from build123d import *

# Parameters (mm, degrees)
SKETCH1_R               = 15
SKETCH1_R_2             = 3
BOSS_EXTRUDE1_DEPTH     = 10
SKETCH2_W               = 15
SKETCH2_H               = 30
BOSS_EXTRUDE2_DEPTH     = 10
FILLET1_R               = 15
SKETCH5_W               = 10
SKETCH5_H               = 2
BOSS_EXTRUDE3_DEPTH     = 10
BOSS_EXTRUDE4_START     = -3
SKETCH7_R               = 3
BOSS_EXTRUDE4_DEPTH     = 3
CHAMFER1_SIZE           = 0.7
BOSS_EXTRUDE6_DEPTH     = 10
FILLET4_R               = 2
FILLET2_R               = 10
CUT_EXTRUDE1_DEPTH      = 63.556116013
CUT_EXTRUDE1_DEPTH_BACK = 63.556116013
SKETCH10_R              = 1.25
SKETCH11_R              = 9.5
SKETCH11_R_2            = 6
CUT_EXTRUDE2_DEPTH      = 5


with BuildPart() as part:
    # Sketch1 → Boss-Extrude1 (new body)
    with BuildSketch(Plane.XY):
        Circle(SKETCH1_R)
        Circle(SKETCH1_R_2, mode=Mode.SUBTRACT)
    extrude(amount=BOSS_EXTRUDE1_DEPTH)

    # Sketch2 → Boss-Extrude2 (add)
    with BuildSketch(Plane.XY):
        with Locations((0, 27.990381057)):
            Rectangle(SKETCH2_W, SKETCH2_H)
    extrude(amount=BOSS_EXTRUDE2_DEPTH)

    # Fillet1
    fillet1_edges = [part.edges().sort_by_distance(p)[0] for p in [
        (-7.5, 12.990381057, 5),
        (7.5, 12.990381057, 5),
    ]]
    fillet(fillet1_edges, radius=FILLET1_R)

    # Sketch5 → Boss-Extrude3 (add)
    with BuildSketch(Plane(origin=(0, 0, 0), x_dir=(-1, 0, 0), z_dir=(0, 0, -1))):
        with Locations((0, 2.5)):
            Rectangle(SKETCH5_W, SKETCH5_H)
    extrude(amount=-BOSS_EXTRUDE3_DEPTH)

    # Sketch7 → Boss-Extrude4 (add)
    with BuildSketch(Plane.XY.offset(10).offset(BOSS_EXTRUDE4_START)):
        Circle(SKETCH7_R)
    extrude(amount=BOSS_EXTRUDE4_DEPTH)

    # Chamfer1
    chamfer1_edges = [part.edges().sort_by_distance(p)[0] for p in [
        (0, 1.5, 7),
        (0, -3, 7),
    ]]
    chamfer(chamfer1_edges, length=CHAMFER1_SIZE)

    # Sketch9 → Boss-Extrude6 (add)
    with BuildSketch(Plane(origin=(0, 0, 0), x_dir=(-1, 0, 0), z_dir=(0, 0, -1))):
        with BuildLine():
            Line((-15, 53.990381057), (-15, 50.490381057))
            ThreePointArc((-15, 50.490381057), (-12.803300859, 45.187080198), (-7.5, 42.990381057))
            Line((-7.5, 42.990381057), (0, 42.990381057))
            Line((0, 42.990381057), (0, 46.490381057))
            Line((0, 46.490381057), (-7.5, 46.490381057))
            ThreePointArc((-7.5, 46.490381057), (-10.328427125, 47.661953932), (-11.5, 50.490381057))
            Line((-11.5, 50.490381057), (-11.5, 53.990381057))
            Line((-11.5, 53.990381057), (-15, 53.990381057))
        make_face()
        with BuildLine():
            Line((0, 46.490381057), (0, 42.990381057))
            Line((0, 42.990381057), (7.5, 42.990381057))
            ThreePointArc((7.5, 42.990381057), (12.803300859, 45.187080198), (15, 50.490381057))
            Line((15, 50.490381057), (15, 53.990381057))
            Line((15, 53.990381057), (11.5, 53.990381057))
            Line((11.5, 53.990381057), (11.5, 50.490381057))
            ThreePointArc((11.5, 50.490381057), (10.328427125, 47.661953932), (7.5, 46.490381057))
            Line((7.5, 46.490381057), (0, 46.490381057))
        make_face()
    extrude(amount=-BOSS_EXTRUDE6_DEPTH)

    # Fillet4
    # the kernel refuses this fillet: 2 mm, written as the material it takes off along each edge
    with BuildSketch(Plane(origin=(11.5, 53.990381057, -5), x_dir=(0, -1, 0), z_dir=(0, 0, 1)), Plane(origin=(15, 53.990381057, -5), x_dir=(-1, 0, 0), z_dir=(0, 0, 1)), Plane(origin=(-11.5, 53.990381057, -5), x_dir=(-1, 0, 0), z_dir=(0, 0, 1)), Plane(origin=(-15, 53.990381057, -5), x_dir=(0, -1, 0), z_dir=(0, 0, 1))) as fillet4_piece_1:
        with BuildLine():
            CenterArc((FILLET4_R, FILLET4_R), FILLET4_R, 180, 90)
            Line((0, FILLET4_R), (0, 0))
            Line((0, 0), (FILLET4_R, 0))
        make_face()
    extrude(amount=20, mode=Mode.SUBTRACT)

    # Fillet2
    fillet2_edges = [part.edges().sort_by_distance(p)[0] for p in [
        (-7.5, 42.990381057, 5),
        (7.5, 42.990381057, 5),
    ]]
    fillet(fillet2_edges, radius=FILLET2_R)

    # Sketch10 → Cut-Extrude1 (cut, two sides: drawn at the far end of the back side and taken through both)
    with BuildSketch(Plane(origin=(15, 0, 0), x_dir=(0, 0, -1), z_dir=(1, 0, 0)).offset(-CUT_EXTRUDE1_DEPTH_BACK)):
        with Locations((-5, 50.490381057)):
            Circle(SKETCH10_R)
    extrude(amount=CUT_EXTRUDE1_DEPTH + CUT_EXTRUDE1_DEPTH_BACK, mode=Mode.SUBTRACT)

    # Sketch11 → Cut-Extrude2 (cut)
    with BuildSketch(Plane.XY.offset(10)):
        Circle(SKETCH11_R)
        Circle(SKETCH11_R_2, mode=Mode.SUBTRACT)
    extrude(amount=-CUT_EXTRUDE2_DEPTH, mode=Mode.SUBTRACT)


solid = part.part
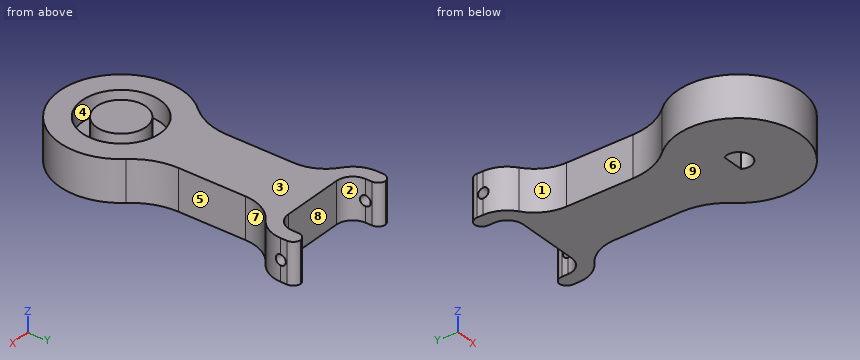
Could you check a few things on this model? Use its own coordinates, in mm. Face numbers are marked on the shaded views. A direction names the side the tool comes from. Give positions to 0.01 mm unless a question says otherwise; leave off trailing zeros. Write each loop counter-clockwise with the first axis right and the second up, starting at its lowest first coordinate (ties: lowest second). Pieces come first, ordered by that corner, then holes. Notation, with made-up numbers: (27.5, -5.75) - (84.5, -5.75) arc R7 ccw to (84.5, 4.25) - close; hole circle Ø5 at (-23.5, 39.25). An arc over 180 degrees is marked (long way). Use CSV: the item, a comma, the result in double quotes. Start each with the question number.
Item 1: I want a section at A-A, the plane z = 3. Please give me the cut outline in (x, y), then the cut area to 3 significant figures.
Item 2: If we mould it in two halves opening along X, with no side actions, what happens to the marked faces 6, 7, 8 and 9? For each: pulls with the +X half, pulls with the -X half, needs draft (parallel to the pull), parting line crosses it, or undercut.
Item 3: I'm going to push flat-ended pins straight in: pin 1 (3 mm diameter, centred on x = -8.5, z = 2.5, fed in from +Y); pin 2 (1.5 mm diameter, centred on x = -0.5, y = -1.5, fed in from -Z); pin 3 (6 mm diameter, centred on x = -4, z = 6, fed in from -Y). Where does each tip first touch, or does it pass through?
Item 4: If I drill on line 1 along Y through (x, z) = (0, 7.9); line 2 along X through (y, z) = (1.5, 8.25); line 3 along Y through (x, z) = (-12.15, 5), over which ranges is the centre line in solid material (lowest first)?
Item 5: I want a section at C-C, the plane x = 0. Please give me the cut outline in (y, z), then the cut area to 3 significant figures.
Item 6: I want a section at B-B, the plane y = 0. Please give me the cut outline in (x, z).
Item 7: For the marked faces 1, 2, 3, 4 and 5, which set-ups out of +Z, -Z, +X, -X, +Y, -Y let a thin tool reach every point of the face, with its end or its side?
Item 8: I want a section at D-D, the plane y = 11. Please give me the cut outline in (x, z), then the cut area to 3 significant figures.
Findings:
1,outline,"(-15, 50.49) arc R7.5 ccw to (-11.79, 44.34) arc R10 cw to (-7.5, 36.13) - (-7.5, 19.84) arc R15 cw to (-11.25, 9.92) arc R15 ccw (long way) to (11.25, 9.92) arc R15 cw to (7.5, 19.84) - (7.5, 36.13) arc R10 cw to (11.79, 44.34) arc R7.5 ccw to (15, 50.49) - (15, 51.99) arc R2 ccw to (13.25, 53.97) arc R2 ccw to (11.5, 51.99) - (11.5, 50.49) arc R4 cw to (7.5, 46.49) - (-7.5, 46.49) arc R4 cw to (-11.5, 50.49) - (-11.5, 51.99) arc R2 ccw to (-13.25, 53.97) arc R2 ccw to (-15, 51.99) - close; hole (-2.6, 1.5) arc R3 ccw (long way) to (2.6, 1.5) - close"
1,area,"1,270 mm2"
2,face 6,"pulls with the -X half"
2,face 7,"pulls with the +X half"
2,face 8,"undercut"
2,face 9,"needs draft"
3,pin 1,"stops at y = 47.37"
3,pin 2,"stops at z = 6.97"
3,pin 3,"stops at y = -14.97"
4,line 1,"y = -15 to -9.5, -6 to 6, 9.5 to 46.49"
4,line 2,"x = -14.92 to -9.38, -5.81 to 5.81, 9.38 to 14.92"
4,line 3,"y = -8.8 to 8.8, 44.61 to 49.24, 51.74 to 53.47"
5,outline,"(-15, 0) - (-3, 0) - (-3, 6.3) - (-2.3, 7) - (0.8, 7) - (1.5, 6.3) - (1.5, 0) - (46.49, 0) - (46.49, 10) - (9.5, 10) - (9.5, 5) - (6, 5) - (6, 10) - (-6, 10) - (-6, 5) - (-9.5, 5) - (-9.5, 10) - (-15, 10) - close"
5,area,"549 mm2"
6,outline,"(-15, 0) - (-3, 0) - (-3, 6.3) - (-2.3, 7) - (2.3, 7) - (3, 6.3) - (3, 0) - (15, 0) - (15, 10) - (9.5, 10) - (9.5, 5) - (6, 5) - (6, 10) - (-6, 10) - (-6, 5) - (-9.5, 5) - (-9.5, 10) - (-15, 10) - close"
7,face 1,"+Z, -Z, -X"
7,face 2,"+Z, -Z, +Y"
7,face 3,"+Z, +X, -X, +Y, -Y"
7,face 4,"+Z"
7,face 5,"+Z, -Z, +X"
8,outline,"(-10.38, 0) - (10.38, 0) - (10.38, 10) - (-10.38, 10) - close"
8,area,"208 mm2"
